Source: CAD feature listing. Evaluate the final solid. Frame: model axes, mm. A direction names the side the tool comes from. Round coordinates to 2 decimals unless told otherwise and drop trailing zeros. Write each loop counter-clockwise with the first axis right and the second up, starting at its lowest first coordinate (ties: lowest second). Pieces come first, ordered by that corner, then holes. Notation, with made-up numbers: (-23.75, -28) -> (-14.75, -28) arc R13 ccw to (-14.75, -6) -> close; hole circle Ø4 at (85, 43). An arc over 180 degrees is marked (long way). Return JSON: item names as keys, results as strings. Group by question number.
Autodesk Fusion 360 part; units mm, degrees
sketch "Sketch1" plane through (0, 0, 0) normal (0, 1, 0) x (1, 0, 0)
  line L0 (0, 0) -> (0, -55)
  line L1 (0, -55) -> (-9.675, -55)
  line L2 (-9.675, -55) -> (-9.675, 0)
  line L3 (-9.675, 0) -> (0, 0)
  line L4 (-7.5, -55) -> (-7.5, -30.5)
  line L5 (-7.5, 0) -> (-7.5, -24.5)
  line L6 (-7.5, -24.5) -> (0, -24.5)
  line L7 (-7.5, -30.5) -> (0, -30.5)
  line L8 (-7.5, -24.5) -> (-7.5, -30.5)
  line L9 (-5.5, -24.5) -> (-5.5, -30.5)
  dimension "d1" = 19.35
  dimension "d2" = 55
  dimension "d5" = 24.5
  dimension "d6" = 24.5
  dimension "d7" = 15
  dimension "d27" = 2
revolve "Revolve1" add sketch "Sketch1" angle 360 about axis through (0, 0, 0) along (0, 0, 1) contours L1 L2 L3 L4 L5 L8 | L6 L7 L8 L9
move_face "OffsetFaces2" offset -0.075 3 faces at (-7.4627, 0.7468, 46.8333) (-7.4907, 0.3738, 16.3333) (-5.4932, 0.2742, 26.5)
chamfer "Chamfer5" distance 0.4 angle 45 2 edges at (7.0624, -2.7392, 55) (-9.0203, 3.4986, 55)
chamfer "Chamfer6" distance 0.2 angle 45 2 edges at (7.0624, -2.7392, 0) (-9.0203, 3.4986, 0)
chamfer "Chamfer7" distance 2 angle 45 2 edges at (5.1977, -2.016, 24.5) (5.1977, -2.016, 30.5)
equation "d6 = d5"
equation "tolerance = ( 0.15 / 2 ) * 1 mm"
Item 1: First-contact query: pin 1 Ø8 at (y, z) = (-6, 30) entering from -X; pin 2 Ø5 at (x, z) = (-7, 11) entering from -Y; pin 3 Ø1.5 at (y, z) = (2.5, 40) entering from +X. Flat tips, straight axial feed; report the tip coordinate or a pass-through.
Item 2: Set-up query: faces 4 (the cylindrical face through (6.01, -4.61, 42.38)), 5 (the cylindrical face through (6.01, 4.61, 12.52)), 6 (the flat face through (-3, -8, 55)). Return all of +Z, -Z, +X, -X, +Y, -Y with unobstructed straight access to the full face (end or side cutting, diameter ignored); none if empty.
Item 3: Material intervals for probe 1 along Y at (x, z) = (0, 36.25) (3 decimals); probe 2 along Y at (x, z) = (0, 27.15) (3 decimals); probe 3 along X at (y, z) = (0.5, 31), sorted ascending.
Item 4: Pull-direction query (Y, two-part tool) for faces 1 (the cylindrical face through (-5.32, -1.67, 27.51)), 2 (the cylindrical face through (9.666, 0.425, 27.019)), 3 (the flat face through (1, -8, 0)); classes: +Y half, -Y half, draft (parallel to the pull), parting line (faces both ways), or undercut.
Item 5: Cut plane C-C on z = 41. Output: boundary loops of the cut face in (x, y) (3 decimals), and give its area (3 significant figures).
Here are the results:
{
 "1": {"pin 1": "stops at x = -9.47", "pin 2": "stops at y = -8.56", "pin 3": "stops at x = 9.52"},
 "2": {"face 4": "+Z", "face 5": "-Z", "face 6": "+Z, +X, -X, +Y, -Y"},
 "3": {"probe 1": "y = -9.675 to -7.575, 7.575 to 9.675", "probe 2": "y = -9.675 to -5.575, 5.575 to 9.675", "probe 3": "x = -9.66 to -7.56, 7.56 to 9.66"},
 "4": {"face 1": "undercut", "face 2": "parting line", "face 3": "draft"},
 "5": {"outline": "circle Ø19.35 at (0, 0); hole circle Ø15.15 at (0, 0)", "area": "114 mm^2"}
}
